Design review of the part built by this model. Coordinates are the model's own, in mm. Face numbers are marked on the shaded views. A direction names the side the tool comes from. Give positions to 0.01 mm unless a question says otherwise; leave off trailing zeros. Loops run counter-clockwise (first coordinate to the right, second up) from the corner with the lowest first, then second, coordinate; pieces in that order, holes last.
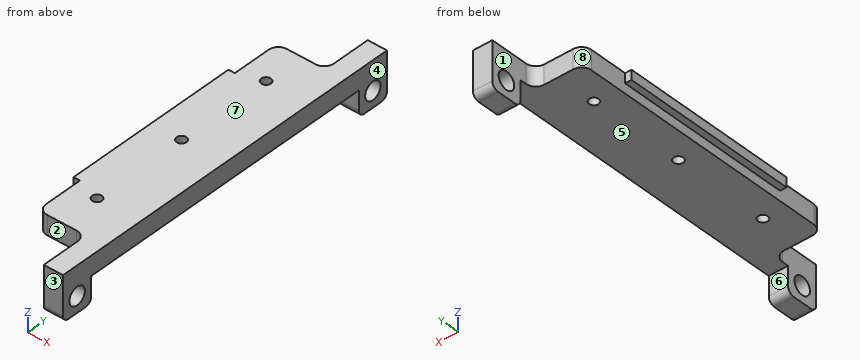
Solid Edge part; units mm, degrees
sketch "Sketch1" plane through (0, 0, 0) normal (0, 0, 1) x (1, 0, 0)
  arc A0 (4.5, 42.5) -> (7.5, 45.5) centre (4.5, 45.5) ccw
  line L0 (7.5, 45.5) -> (7.5, 57.5)
  line L1 (7.5, 57.5) -> (13.5, 57.5)
  line L2 (13.5, 57.5) -> (13.5, -57.5)
  line L3 (13.5, -57.5) -> (7.5, -57.5)
  line L4 (7.5, -57.5) -> (7.5, -45.5)
  arc A1 (4.5, -42.5) -> (7.5, -45.5) centre (4.5, -45.5) cw
  line L5 (-7.5, -42.5) -> (4.5, -42.5)
  line L6 (-7.5, 42.5) -> (-7.5, -42.5)
  line L7 (4.5, 42.5) -> (-7.5, 42.5)
  circle A2 centre (0, 0) radius 1.5
  circle A3 centre (0, -30) radius 1.5
  circle A4 centre (0, 30) radius 1.5
extrude "Protrusion1" add sketch "Sketch1" along normal blind 6
fillet "Round_1" radius 3 2 edges at (-7.5, 42.5, 3) (-7.5, -42.5, 3)
sketch "Sketch2" plane through (13.5, 0, 2) normal (1, 0, 0) x (0, 1, 0)
  line L0 (-57.5, -2) -> (-47.5, -2)
  line L1 (-47.5, -2) -> (-47.5, -8)
  arc A0 (-49.5, -10) -> (-47.5, -8) centre (-49.5, -8) ccw
  line L2 (-49.5, -10) -> (-55.5, -10)
  arc A1 (-55.5, -10) -> (-57.5, -8) centre (-55.5, -8) cw
  line L3 (-57.5, -8) -> (-57.5, -2)
  circle A2 centre (-52.5, -5) radius 1.75
  line L4 (57.5, -2) -> (47.5, -2)
  line L5 (47.5, -2) -> (47.5, -8)
  arc A3 (49.5, -10) -> (47.5, -8) centre (49.5, -8) cw
  line L6 (49.5, -10) -> (55.5, -10)
  arc A4 (55.5, -10) -> (57.5, -8) centre (55.5, -8) ccw
  line L7 (57.5, -8) -> (57.5, -2)
  circle A5 centre (52.5, -5) radius 1.75
extrude "ExtrudedProtrusion_2" add sketch "Sketch2" against normal blind 6
sketch "Sketch3" plane through (-7.5, 0, 3) normal (-1, 0, 0) x (0, -1, 0)
  line L0 (-27.5, 0) -> (27.5, 0)
  line L1 (27.5, 0) -> (27.5, 3)
  line L2 (27.5, 3) -> (-27.5, 3)
  line L3 (-27.5, 3) -> (-27.5, 0)
extrude "ExtrudedProtrusion_3" add sketch "Sketch3" along normal blind 2
sketch "Sketch4" plane through (13.5, 0, -1) normal (1, 0, 0) x (0, 1, 0)
  circle A0 centre (-52.5, -2) radius 2.75
  circle A1 centre (52.5, -2) radius 2.75
extrude "ExtrudedCutout_1" cut sketch "Sketch4" against normal blind 10
Q1. Take a section at C-C (x = 0). Give the boundary of the cut face in (y, z).
Results:
outline: (-42.5, 0) - (-31.5, 0) - (-31.5, 6) - (-42.5, 6) - close; (-28.5, 0) - (-1.5, 0) - (-1.5, 6) - (-28.5, 6) - close; (1.5, 0) - (28.5, 0) - (28.5, 6) - (1.5, 6) - close; (31.5, 0) - (42.5, 0) - (42.5, 6) - (31.5, 6) - close
Q2. Draft analysis for pull direction Y (two halves, no side actions). For the marked faces 6, 7 and 8, state which applies: pulls with the +Y half, pulls with the -Y half, needs draft (parallel to the pull), parting line crosses it, or undercut.
Results:
face 6: undercut
face 7: needs draft
face 8: pulls with the +Y half
Q3. Tool access review of the marked faces 1, 2, 3, 4 and 5: name each direction out of +Z, -Z, +X, -X, +Y, -Y from which nothing blocks a thin tool from reaching the whole face with its end or side.
Results:
face 1: +Z, -Z, -X, +Y
face 2: +Z, -Z, -X, -Y
face 3: +Z, -Z, +X, -X, -Y
face 4: +Z, -Z, +X, +Y, -Y
face 5: -Z, +X, -X
Q4. Take a section at A-A (x = 10.5). Give the boundary of the cut face in (y, z), plus the area to 3 significant figures.
Results:
outline: (-57.5, -6) arc R2 ccw to (-55.5, -8) - (-49.5, -8) arc R2 ccw to (-47.5, -6) - (-47.5, 0) - (47.5, 0) - (47.5, -6) arc R2 ccw to (49.5, -8) - (55.5, -8) arc R2 ccw to (57.5, -6) - (57.5, 6) - (-57.5, 6) - close; hole circle Ø5.5 at (-52.5, -3); hole circle Ø5.5 at (52.5, -3)
area: 799 mm2
Q5. Wall thickness on line 1 (Y direction, x = 0, z = 2.85); line 2 (Y direction, x = 12.5, z = -3.25); line 3 (Z direction, x = 11, y = 52.5): over which ranges is each line inside the solid? List them lowest first.
Results:
line 1: y = -42.5 to -31.5, -28.5 to -1.5, 1.5 to 28.5, 31.5 to 42.5
line 2: y = -57.5 to -55.24, -49.76 to -47.5, 47.5 to 49.76, 55.24 to 57.5
line 3: z = -8 to -5.75, -0.25 to 6
Q6. Take a section at D-D (y = 14). Give the boundary of the cut face in (x, z).
Results:
outline: (-9.5, 3) - (-7.5, 3) - (-7.5, 0) - (13.5, 0) - (13.5, 6) - (-9.5, 6) - close
Q7. Take a section at B-B (y = 52.5). Give the boundary of the cut face in (x, z).
Results:
outline: (7.5, -8) - (13.5, -8) - (13.5, -5.75) - (7.5, -5.75) - close; (7.5, -0.25) - (13.5, -0.25) - (13.5, 6) - (7.5, 6) - close
Q8. Insertion check: pin 1 (6.5 mm diameter, centred on x = 1.5, z = 3.5, fed in from +Y); pin 2 (4.5 mm diameter, centred on y = -52.5, z = -3, fed in from -X); pin 3 (10.5 mm diameter, centred on x = -1, y = 2.5, fed in from -Z); pin 4 (2 mm diameter, centred on x = -9, z = 4.5, fed in from -Y). Each pin has a flat end and moves straight along its axis. Give the tip position at first contact, or say it passes through.
Results:
pin 1: stops at y = 42.51
pin 2: passes through
pin 3: stops at z = 0
pin 4: stops at y = -27.5
